The drawing under review shows one solid part. Ordinate dimensions are in mm from its lowest x, y, z. A direction names the side the tool comes from. Round coordinates to 2 decimals unless told otherwise and drop trailing zeros. Write each loop counter-clockwise with the first axis right and the second up, starting at its lowest first coordinate (ties: lowest second). Pieces come first, ordered by that corner, then holes. Notation, with made-up numbers: (21, -11.5) -> (63, -11.5) arc R25 cw to (63, 0.5) -> close; hole circle Ø11 at (-6, 44). An arc over 180 degrees is marked (long way). Answer in a Markdown table with one row per item.
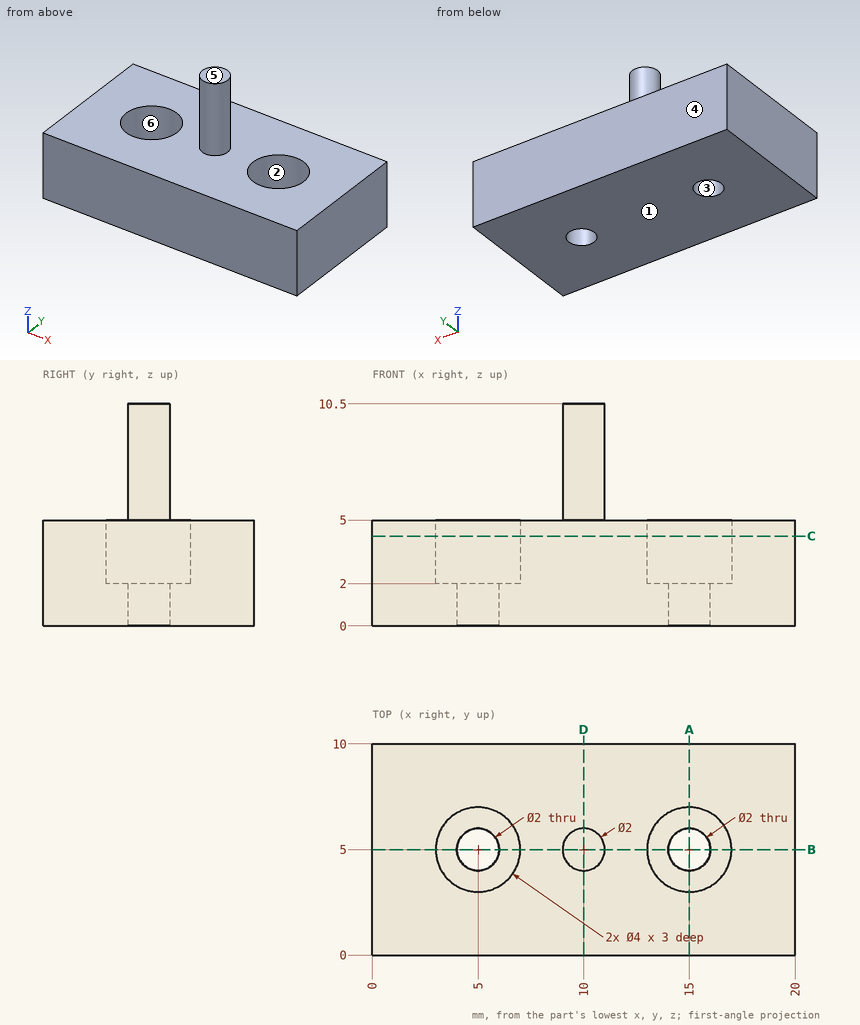
1) Clearance check with flat-ended pins moving along their axes: pin 1 Ø3 at (x, y) = (4.5, 4.5) entering from +Z; pin 2 Ø1.2 at (x, y) = (15, 5.5) entering from +Z. State where each tip first meets the part, or that it passes through.
Solved:
| item | result |
|---|---|
| pin 1 | z = 5 |
| pin 2 | z = 2 |
2) Consider section C-C on z = 4.25. State the section outline as (x, y) points, then the cut area to 3 significant figures.
Solved:
| item | result |
|---|---|
| outline | (0, 0) -> (20, 0) -> (20, 10) -> (0, 10) -> close; hole circle Ø4 at (5, 5); hole circle Ø4 at (15, 5) |
| area | 175 mm² |
3) For line 1 (X direction, y = 5, z = 0.4); line 2 (Y direction, x = 5, z = 0.7); line 3 (Y direction, x = 5, z = 3.65), list the stretches that pass through material, from the lowest coordinate up. Write a range as [from, to].
Solved:
| item | result |
|---|---|
| line 1 | [0, 4], [6, 14], [16, 20] |
| line 2 | [0, 4], [6, 10] |
| line 3 | [0, 3], [7, 10] |
4) Consider section A-A on x = 15. State the section outline as (y, z) points.
Solved:
| item | result |
|---|---|
| outline | (0, 0) -> (4, 0) -> (4, 2) -> (3, 2) -> (3, 5) -> (0, 5) -> close; (6, 0) -> (10, 0) -> (10, 5) -> (7, 5) -> (7, 2) -> (6, 2) -> close |
5) Consider section B-B on y = 5. State the section outline as (x, z) points.
Solved:
| item | result |
|---|---|
| outline | (0, 0) -> (4, 0) -> (4, 2) -> (3, 2) -> (3, 5) -> (0, 5) -> close; (6, 0) -> (14, 0) -> (14, 2) -> (13, 2) -> (13, 5) -> (11, 5) -> (11, 10.5) -> (9, 10.5) -> (9, 5) -> (7, 5) -> (7, 2) -> (6, 2) -> close; (16, 0) -> (20, 0) -> (20, 5) -> (17, 5) -> (17, 2) -> (16, 2) -> close |
6) Consider section D-D on x = 10. State the section outline as (y, z) points.
Solved:
| item | result |
|---|---|
| outline | (0, 0) -> (10, 0) -> (10, 5) -> (6, 5) -> (6, 10.5) -> (4, 10.5) -> (4, 5) -> (0, 5) -> close |
7) For the marked faces 1 and 2, list the 3-axis set-ups (+Z, -Z, +X, -X, +Y, -Y) from which the entire face can be reached by the end or side of a thin tool; tool diameter is ignored.
Solved:
| item | result |
|---|---|
| face 1 | -Z, +X, -X, +Y, -Y |
| face 2 | +Z |
8) Mouldability with a two-part tool opening along Y and no side actions: class the marked faces 3, 4, 5 and 6 as pulls with the +Y half, pulls with the -Y half, needs draft (parallel to the pull), parting line crosses it, or undercut.
Solved:
| item | result |
|---|---|
| face 3 | undercut |
| face 4 | pulls with the +Y half |
| face 5 | needs draft |
| face 6 | undercut |
